from build123d import *

# Parameters (mm, degrees)
SKETCH1_W              = 76.2
SKETCH1_H              = 82
BOSS_EXTRUDE1_DEPTH    = 3.175
CUT_EXTRUDE2_DEPTH     = 57.328789264
M3_5_CLEARANCE_HOLE1_D = 3.9
CUT_EXTRUDE6_DEPTH     = 57.328789264
CUT_EXTRUDE7_DEPTH     = 57.328789264
CIRPATTERN1_COUNT      = 4


with BuildPart() as part:
    # Sketch1 → Boss-Extrude1 (new, symmetric)
    with BuildSketch(Plane(origin=(0, 0, 0), x_dir=(1, 0, 0), z_dir=(0, 1, 0))):
        Rectangle(SKETCH1_W, SKETCH1_H)
    extrude(amount=BOSS_EXTRUDE1_DEPTH, both=True)

    # Sketch8 → Cut-Extrude2 (cut, through all)
    with BuildSketch(Plane(origin=(0, 3.175, 0), x_dir=(1, 0, 0), z_dir=(0, 1, 0))):
        with BuildLine():
            Line((-33.8582, -17.1875), (-33.8582, -14.0125))
            ThreePointArc((-33.8582, -14.0125), (-30.48, -10.6343), (-27.1018, -14.0125))
            Line((-27.1018, -14.0125), (-27.1018, -17.1875))
            ThreePointArc((-27.1018, -17.1875), (-30.48, -20.5657), (-33.8582, -17.1875))
        make_face()
        with BuildLine():
            Line((-33.8582, 20.9125), (-33.8582, 24.0875))
            ThreePointArc((-33.8582, 24.0875), (-30.48, 27.4657), (-27.1018, 24.0875))
            Line((-27.1018, 24.0875), (-27.1018, 20.9125))
            ThreePointArc((-27.1018, 20.9125), (-30.48, 17.5343), (-33.8582, 20.9125))
        make_face()
    cut_extrude2 = extrude(amount=-CUT_EXTRUDE2_DEPTH, mode=Mode.SUBTRACT)

    # Mirror1: Cut-Extrude2 across plane
    add(cut_extrude2.mirror(Plane(origin=(0, 0, 0), x_dir=(0, 0, 1), z_dir=(1, 0, 0))), mode=Mode.SUBTRACT)

    # M3.5 Clearance Hole1 (through all)
    with Locations(Plane(origin=(0, 3.175, 0), x_dir=(1, 0, 0), z_dir=(0, 1, 0))):
        with Locations((-15.5, 2.951), (15.5, 2.951), (15.5, -28.049), (-15.5, -28.049)):
            Hole(M3_5_CLEARANCE_HOLE1_D / 2)

    # Sketch23 → Cut-Extrude6 (cut, through all)
    with BuildSketch(Plane(origin=(0, 3.175, 0), x_dir=(1, 0, 0), z_dir=(0, 1, 0))):
        with BuildLine():
            Line((-12.9860741, 8.471), (-12.9860741, 4.551180167))
            ThreePointArc((-12.9860741, 4.551180167), (-13.392821792, 0.843821792), (-17.100180167, 0.4370741))
            Line((-17.100180167, 0.4370741), (-21.02, 0.4370741))
            Line((-21.02, 0.4370741), (-21.02, -25.5350741))
            Line((-21.02, -25.5350741), (-17.100180167, -25.5350741))
            ThreePointArc((-17.100180167, -25.5350741), (-13.392821792, -25.941821792), (-12.9860741, -29.649180167))
            Line((-12.9860741, -29.649180167), (-12.9860741, -33.569))
            Line((-12.9860741, -33.569), (12.9860741, -33.569))
            Line((12.9860741, -33.569), (12.9860741, -29.649180167))
            ThreePointArc((12.9860741, -29.649180167), (13.392821792, -25.941821792), (17.100180167, -25.5350741))
            Line((17.100180167, -25.5350741), (21.02, -25.5350741))
            Line((21.02, -25.5350741), (21.02, 0.4370741))
            Line((21.02, 0.4370741), (17.100180167, 0.4370741))
            ThreePointArc((17.100180167, 0.4370741), (13.392821792, 0.843821792), (12.9860741, 4.551180167))
            Line((12.9860741, 4.551180167), (12.9860741, 8.471))
            Line((12.9860741, 8.471), (-12.9860741, 8.471))
        make_face()
    extrude(amount=-CUT_EXTRUDE6_DEPTH, mode=Mode.SUBTRACT)

    # Sketch24 → Cut-Extrude7 (cut, through all)
    with BuildSketch(Plane(origin=(0, 3.175, 0), x_dir=(1, 0, 0), z_dir=(0, 1, 0))):
        with BuildLine():
            Line((-18.979586404, 0.984476566), (-19.479586404, 0.984476566))
            ThreePointArc((-19.479586404, 0.984476566), (-21.954460139, -0.0406497), (-22.979586404, -2.515523434))
            Line((-22.979586404, -2.515523434), (-22.979586404, -22.582476566))
            ThreePointArc((-22.979586404, -22.582476566), (-21.954460139, -25.0573503), (-19.479586404, -26.082476566))
            Line((-19.479586404, -26.082476566), (-18.979586404, -26.082476566))
            ThreePointArc((-18.979586404, -26.082476566), (-18.000834998, -25.942840487), (-17.100180167, -25.5350741))
            ThreePointArc((-17.100180167, -25.5350741), (-13.392821792, -25.941821792), (-12.9860741, -29.649180167))
            Line((-12.9860741, -29.649180167), (-7.9860741, -29.649180167))
            Line((-7.9860741, -29.649180167), (-7.9860741, 4.551180167))
            Line((-7.9860741, 4.551180167), (-12.9860741, 4.551180167))
            ThreePointArc((-12.9860741, 4.551180167), (-13.392821792, 0.843821792), (-17.100180167, 0.4370741))
            ThreePointArc((-17.100180167, 0.4370741), (-18.000834998, 0.844840487), (-18.979586404, 0.984476566))
        make_face()
    cut_extrude7 = extrude(amount=-CUT_EXTRUDE7_DEPTH, mode=Mode.SUBTRACT)

    # CirPattern1: Cut-Extrude7 ×4 about axis
    cirpattern1_axis = Axis((0, 0, 12.549), (0, 1, 0))
    for i in range(1, CIRPATTERN1_COUNT):
        add(cut_extrude7.rotate(cirpattern1_axis, i * 360 / CIRPATTERN1_COUNT), mode=Mode.SUBTRACT)


solid = part.part
Read the model definition and answer for the solid it produces. Units are mm, in the model's axes. Coordinates: 2 decimals unless noted, no trailing zeros. Order: outer loops, then holes, each group sorted by start corner. A loop starts at its lowest first (then second) coordinate and runs counter-clockwise, first axis right, second up. Notation, with made-up numbers: M 89.25,44.25 L 121.25,44.25 A16 cw 121.25,61.25 Z; hole C 77.5,47 d1. An arc over 180 degrees is marked long. Put each result on its own line as item: value. Start each with the question number.
Item 1: The mould has two halves that part along X. Classify faces 1 (the face through (21.982, 0.044, 0.068)), 2 (the face through (38.1, 0, 1)), 3 (the face through (22.98, 0, 13)): +X half, -X half, draft (parallel to the pull), parting line (faces both ways), or undercut.
Item 2: Given pin 1 Ø8 at (x, z) = (16.5, 18.5) entering from -Y, flat-ended and moving along its own axis, determine where the tip first touches the part or whether it passes through.
Item 3: Section A-A, the plane x = 2 is taken. Determine the outline of the cut face in (y, z) (3 decimals).
Item 4: Section B-B, the plane x = -30.48 is taken. Determine the outline of the cut face in (y, z) (3 decimals), plus the area to 3 significant figures.
Item 5: Section C-C, the plane z = -8 is taken. Determine the outline of the cut face in (x, y) (3 decimals), plus the area to 3 significant figures.
Item 6: Consider probe 1 along Z at (x, y) = (-15.5, 1.5); probe 2 along Z at (x, y) = (-5, 2); probe 3 along X at (y, z) = (2.5, 27). Determine where each line is inside the solid, lowest interval first. Write a range as [from, to].
Item 7: Section D-D, the plane x = -15.5 is taken. Determine the outline of the cut face in (y, z) (3 decimals), plus the area to 3 significant figures.
Computed:
1. face 1: undercut
1. face 2: +X half
1. face 3: undercut
2. pin 1: passes through
3. outline: M -3.175,-41 L 3.175,-41 L 3.175,-10.431 L -3.175,-10.431 Z; M -3.175,35.529 L 3.175,35.529 L 3.175,41 L -3.175,41 Z
4. outline: M -3.175,-41 L 3.175,-41 L 3.175,-27.466 L -3.175,-27.466 Z; M -3.175,-17.534 L 3.175,-17.534 L 3.175,10.634 L -3.175,10.634 Z; M -3.175,20.566 L 3.175,20.566 L 3.175,41 L -3.175,41 Z
4. area: 395 mm2
5. outline: M -38.1,-3.175 L -13.366,-3.175 L -13.366,3.175 L -38.1,3.175 Z; M 13.366,-3.175 L 38.1,-3.175 L 38.1,3.175 L 13.366,3.175 Z
5. area: 314 mm2
6. probe 1: z = [-41, -4.9], [-1, 0.03], [25.07, 26.1], [30, 41]
6. probe 2: z = [-41, -10.43], [35.53, 41]
6. probe 3: x = [-38.1, -17.14], [-13.86, -12.71], [12.71, 13.86], [17.14, 38.1]
7. outline: M -3.175,-41 L 3.175,-41 L 3.175,-4.901 L -3.175,-4.901 Z; M -3.175,-1.001 L 3.175,-1.001 L 3.175,0.029 L -3.175,0.029 Z; M -3.175,25.069 L 3.175,25.069 L 3.175,26.099 L -3.175,26.099 Z; M -3.175,29.999 L 3.175,29.999 L 3.175,41 L -3.175,41 Z
7. area: 312 mm2
